Can you work these out from the drawing? Everything is in mm from the part's minimum corner. Give positions to 0.01 mm unless a question says otherwise; leave off trailing zeros. Loops run counter-clockwise (first coordinate to the right, second up) from the corner with the lowest first, then second, coordinate; pieces in that order, holes last.
Q1. If we section it at A-A (x = 11.25): Please give me the cut outline in (y, z).
Q2. I need wall thicknesses on line 1 (Y direction, x = 4.5, z = 8); line 2 (Y direction, x = 4.5, z = 1); line 3 (X direction, y = 8.75, z = 3). Which ranges of each line are inside material? Lowest first, please.
Q3. Will these pins go through, and if not, where does the flat tip stop? P1, Ø1.5, axis at x = 6, y = 2, coming from the +Z side; P2, Ø1, axis at x = 26, y = 8, coming from the +Z side; P3, Ø1.5, axis at x = 13.5, z = 3, coming from the -Y side.
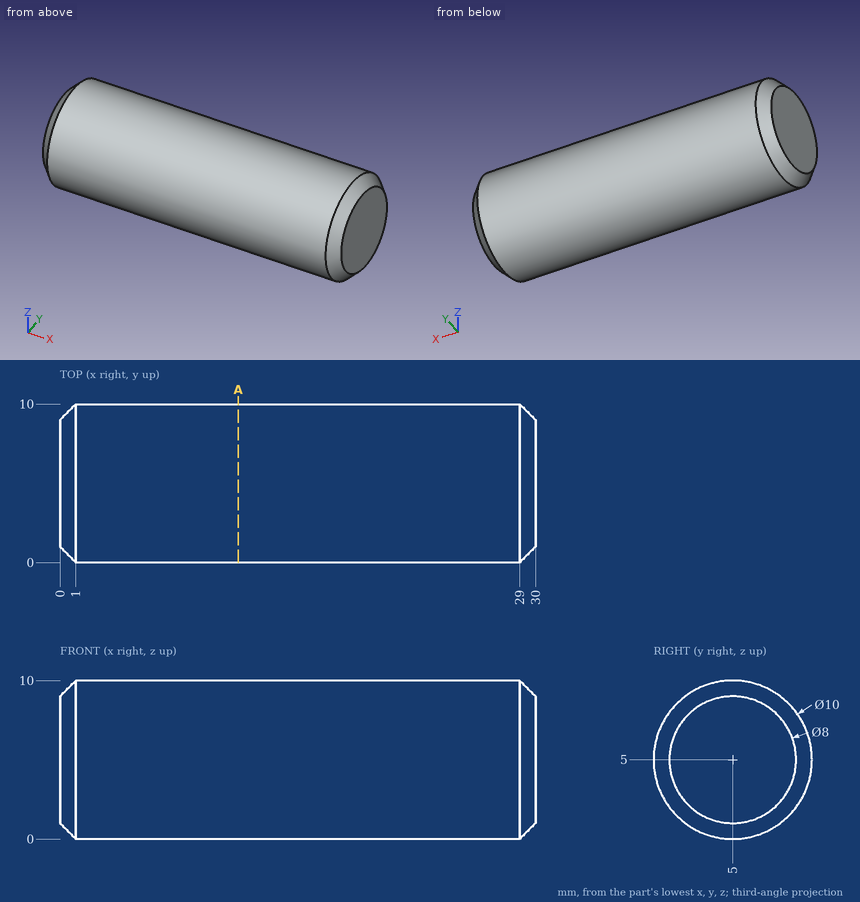
Check sheet entries:
1. outline: circle Ø10 at (5, 5)
2. line 1: y = 1 to 9
2. line 2: y = 2 to 8
2. line 3: x = 0.25 to 29.75
3. P1: stops at z = 9.47
3. P2: stops at z = 9.33
3. P3: stops at y = 0.16
